Here's how the part is built. I have some questions about the finished solid (model axes, mm). Face numbers are marked on the shaded views. A direction names the side the tool comes from. Round coordinates to 2 decimals unless told otherwise and drop trailing zeros. Order: outer loops, then holes, each group sorted by start corner. A loop starts at its lowest first (then second) coordinate and runs counter-clockwise, first axis right, second up. Notation, with made-up numbers: (84.5, 81) -> (140.5, 81) arc R34 ccw to (140.5, 116) -> close; hole circle Ø5 at (25, 33.5). An arc over 180 degrees is marked (long way). Use a Markdown table: item, result. Add a question column.
(1) On a 3-axis mill with a long thin cutter (end or side, diameter ignored), from which of +Z, -Z, +X, -X, +Y, -Y can I reach the whole of each face in a straight line? I mean the marked faces 4, 5 and 6. Say none if no direction works.
(2) I'm going to push flat-ended pins straight in: P1, Ø15, axis at x = 78, z = 30, coming from the -Y side; P2, Ø4, axis at x = 50, y = 37, coming from the +Z side; P3, Ø22.5, axis at y = 39.5, z = 34.5, coming from the +X side. Where does each tip first touch, or does it pass through?
(3) Thinking about a two-plate mould opening in Y: for the marked faces 1, 2 and 3, which applies, pulls with the +Y half, pulls with the -Y half, needs draft (parallel to the pull), parting line crosses it, or undercut?
(4) If I drill on probe 1 along X at (y, z) = (11, 56); probe 2 along X at (y, z) = (42.5, 20); probe 3 along Y at (x, z) = (23, 20), over which ranges is the centre line in solid material (lowest first)?
(5) I want a section at C-C, the plane x = 35. Please give me the cut outline in (y, z).
(6) I want a section at B-B, the plane z = 38. Please give me the cut outline in (x, y), then the cut area to 3 significant figures.
(7) I want a section at A-A, the plane y = 43.5. Please give me the cut outline in (x, z).
(8) I want a section at D-D, the plane x = 12. Please give me the cut outline in (y, z), then the cut area to 3 significant figures.
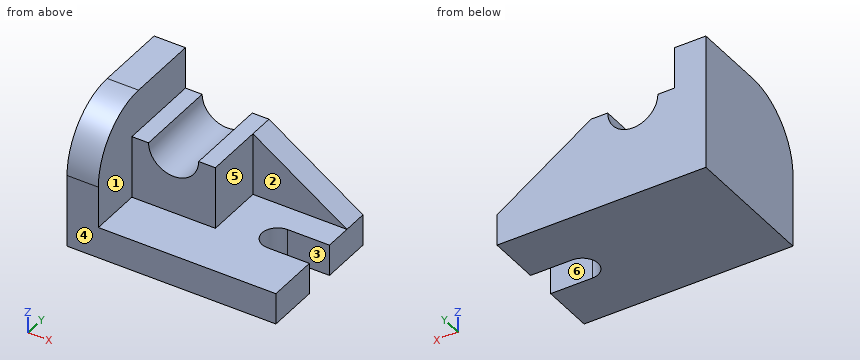
Autodesk Fusion 360 part; units mm, degrees
sketch "Sketch1" plane through (0, 0, 0) normal (0, 0, 1) x (1, 0, 0)
  line L0 (0, 0) -> (100, 0)
  line L1 (100, 0) -> (100, 65)
  line L2 (100, 65) -> (0, 65)
  line L3 (0, 65) -> (0, 0)
  dimension "d1" = 100
  dimension "d2" = 65
extrude "Extrude1" add sketch "Sketch1" along normal blind 15
sketch "Sketch2" plane through (0, 0, 15) normal (0, 0, 1) x (-1, 0, 0)
  line L0 (0, -65) -> (0, 0)
  line L1 (0, 0) -> (-100, 0)
  line L2 (-100, 0) -> (-100, -65)
  line L3 (-100, -65) -> (0, -65)
  line L4 (0, -65) -> (-15, -65)
  line L5 (-15, -65) -> (-15, 0)
  line L6 (-15, 0) -> (0, 0)
  line L7 (0, 0) -> (0, -65)
  line L8 (-15, -65) -> (-55, -65)
  line L9 (-55, -65) -> (-55, -25)
  line L10 (-55, -25) -> (-15, -25)
  line L11 (-15, -25) -> (-15, -65)
  line L12 (-55, -65) -> (-100, -65)
  line L13 (-100, -65) -> (-100, -53)
  line L14 (-100, -53) -> (-55, -53)
  line L15 (-55, -53) -> (-55, -65)
  line L16 (-80, -40) -> (-100, -40)
  line L17 (-100, -40) -> (-100, -25)
  line L18 (-100, -25) -> (-80, -25)
  arc A0 (-80, -40) -> (-80.003, -25) centre (-80, -32.5) ccw
  dimension "d5" = 15
  dimension "d6" = 65
  dimension "d7" = 40
  dimension "d8" = 40
  dimension "d9" = 45
  dimension "d10" = 12
  dimension "d11" = 15
  dimension "d12" = 20
  dimension "d13" = 20
  dimension "d14" = 15
extrude "Extrude2" add sketch "Sketch2" along normal blind 50 contours L0 L1 L3 L4 L5 L6 L7 L11
extrude "Extrude3" add sketch "Sketch2" along normal blind 30 contours L3 L5 L8 L9 L10 L11 L15 | L2 L3 L9 L12 L13 L14 L15
extrude "Extrude4" cut sketch "Sketch2" against normal blind 30 contours L2 L16 L17 L18 A0
sketch "Sketch3" plane through (0, 53, 0) normal (0, -1, 0) x (1, 0, 0)
  line L0 (55, 15) -> (100, 15)
  line L1 (100, 15) -> (100, 45)
  line L2 (100, 45) -> (55, 45)
  line L3 (55, 45) -> (55, 15)
  line L4 (55, 45) -> (100, 15)
  line L5 (100, 45) -> (55, 45)
  line L6 (100, 45) -> (100, 15)
fillet "Fillet1" radius 30 1 edges at (7.5, 0, 65)
sketch "Sketch5" plane through (0, 25, 0) normal (0, -1, 0) x (1, 0, 0)
  line L0 (15, 15) -> (55, 15)
  line L1 (55, 15) -> (55, 45)
  line L2 (55, 45) -> (15, 45)
  line L3 (15, 45) -> (15, 15)
  line L4 (15, 45) -> (23, 45)
  line L5 (55, 45) -> (47, 45)
  line L6 (23, 45) -> (35, 45)
  circle A0 centre (35, 45) radius 12
  dimension "d25" = 8
  dimension "d26" = 8
  dimension "d27" = 12
  dimension "d28" = 24
chamfer "Chamfer1" distance 45 distance2 30 1 edges at (100, 59, 45) measured on face at (28.3333, 47.6667, 45)
sketch "Sketch6" plane through (0, 0, 45) normal (0, 0, 1) x (-1, 0, 0)
  line L0 (-55, -53) -> (-55, -65)
  line L1 (-55, -65) -> (-15, -65)
  line L2 (-15, -65) -> (-15, -25)
  line L3 (-15, -25) -> (-55, -25)
  line L4 (-55, -25) -> (-55, -53)
  line L5 (-35, -65) -> (-47, -65)
  line L6 (-47, -65) -> (-47, -25)
  line L7 (-47, -25) -> (-35, -25)
  line L8 (-35, -25) -> (-35, -65)
  dimension "d33" = 12
  dimension "d34" = 40
revolve "Revolve1" cut sketch "Sketch6" angle 360 about axis through (35, 25, 45) along (0, 1, 0) contours L1 L3 L5 L6 L7 L8
Taken from the geometry:
| question | item | result |
|---|---|---|
| 1 | face 4 | +Z, -Z, +X, -X, -Y |
| 1 | face 5 | +Z, +X, -Y |
| 1 | face 6 | +Z, -Z, +X |
| 2 | P1 | stops at y = 53 |
| 2 | P2 | stops at z = 45 |
| 2 | P3 | stops at x = 55 |
| 3 | face 1 | needs draft |
| 3 | face 2 | pulls with the -Y half |
| 3 | face 3 | undercut |
| 4 | probe 1 | x = 0 to 15 |
| 4 | probe 2 | x = 0 to 55 |
| 4 | probe 3 | y = 25 to 65 |
| 5 | outline | (0, 0) -> (65, 0) -> (65, 33) -> (25, 33) -> (25, 15) -> (0, 15) -> close |
| 6 | outline | (0, 0.15) -> (15, 0.15) -> (15, 25) -> (25.25, 25) -> (25.25, 65) -> (0, 65) -> close; (44.75, 25) -> (55, 25) -> (55, 53) -> (65.5, 53) -> (65.5, 65) -> (44.75, 65) -> close |
| 6 | area | 1,920 mm2 |
| 7 | outline | (0, 0) -> (100, 0) -> (100, 15) -> (55, 15) -> (55, 45) -> (47, 45) arc R12 cw to (23, 45) -> (15, 45) -> (15, 65) -> (0, 65) -> close |
| 8 | outline | (0, 0) -> (65, 0) -> (65, 65) -> (30, 65) arc R30 ccw to (0, 35) -> close |
| 8 | area | 4,030 mm2 |
